Print and shaded views of the part. All mm, measured from the part's lowest x, y and z. A direction names the side the tool comes from. Give positions to 0.01 mm unless a question says otherwise; leave off trailing zeros. Loops run counter-clockwise (first coordinate to the right, second up) from the corner with the lowest first, then second, coordinate; pieces in that order, holes last. Notation, with made-up numbers: (27, 25) -> (56, 25) arc R29 ccw to (56, 57) -> close; hole circle Ø7 at (70.5, -19.5). An arc over 180 degrees is marked (long way). Answer as a JSON object with one key per item and string values. Group by question number.
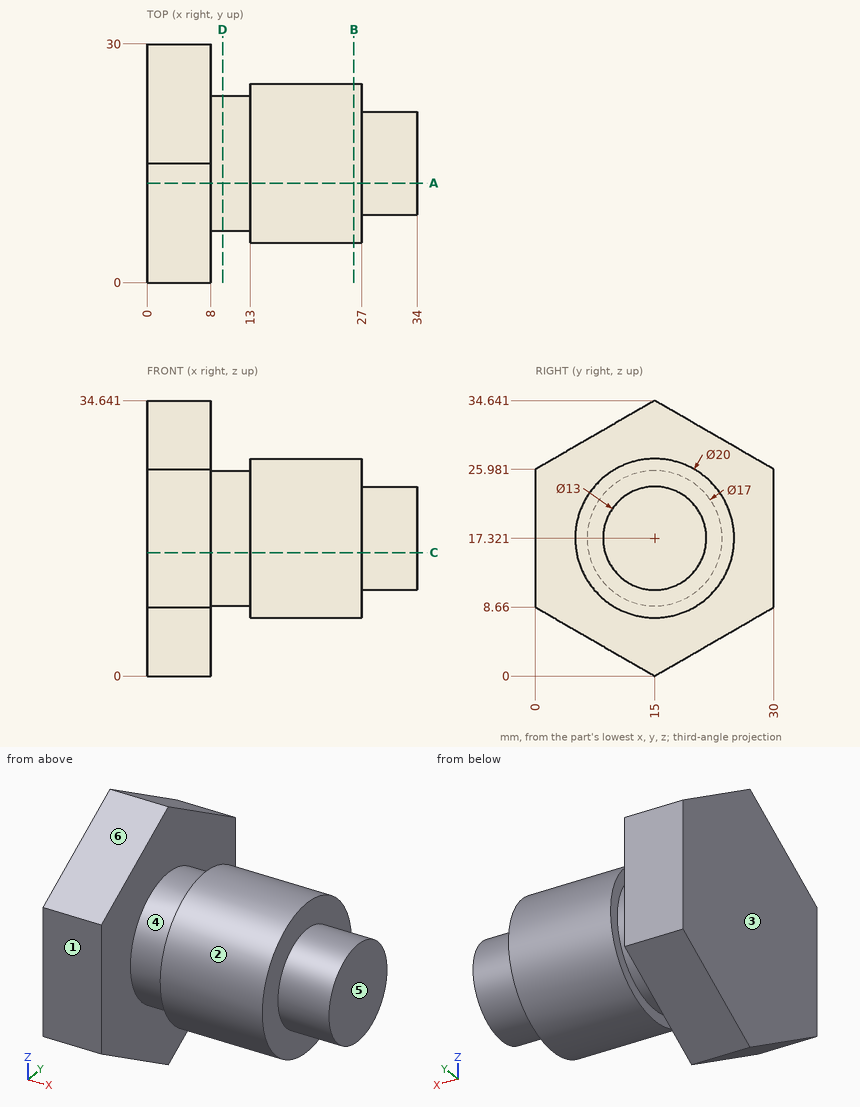
(1) Saw through at A-A on y = 12.5. List the corners of the cut face in (x, z) (1 decimal).
(2) Saw through at C-C on z = 15.5. List the corners of the cut face in (x, y).
(3) Pull direction X, two halves, no side cores. Call the marked faces 3, 4, 5 and 6: pulls with the +X half, pulls with the -X half, needs draft (parallel to the pull), parting line crosses it, or undercut.
(4) Saw through at D-D on x = 9.5. List the corners of the cut face in (y, z), plus the area to 3 significant figures.
(5) 3-axis set-ups, long thin cutter, end or side, ignore diameter. For the marked faces 1 and 2: which of +Z, -Z, +X, -X, +Y, -Y reach the whole face in a straight line?
(6) Probe line 1 along X through (y, z) = (6.5, 21); line 2 along X through (y, z) = (21.75, 16.5); line 3 along X through (y, z) = (15.25, 30.5). List the from-to ranges inside material, lowest first. Write a range as [from, to].
(7) Pin check, flat tips, straight feed: pin 1 (4 mm diameter, centred on y = 15.5, z = 29.5, fed in from +X); pin 2 (1.5 mm diameter, centred on x = 26, y = 21.5, fed in from -Z); pin 3 (2 mm diameter, centred on y = 14, z = 26.5, fed in from +X). Stop position of each tip, or through.
(8) Saw through at B-B on x = 26. List the corners of the cut face in (y, z).
Calculated:
{
 "1": {"outline": "(0, 1.4) -> (8, 1.4) -> (8, 9.2) -> (13, 9.2) -> (13, 7.6) -> (27, 7.6) -> (27, 11.3) -> (34, 11.3) -> (34, 23.3) -> (27, 23.3) -> (27, 27) -> (13, 27) -> (13, 25.4) -> (8, 25.4) -> (8, 33.2) -> (0, 33.2) -> close"},
 "2": {"outline": "(0, 0) -> (8, 0) -> (8, 6.7) -> (13, 6.7) -> (13, 5.17) -> (27, 5.17) -> (27, 8.76) -> (34, 8.76) -> (34, 21.24) -> (27, 21.24) -> (27, 24.83) -> (13, 24.83) -> (13, 23.3) -> (8, 23.3) -> (8, 30) -> (0, 30) -> close"},
 "3": {"face 3": "pulls with the -X half", "face 4": "undercut", "face 5": "pulls with the +X half", "face 6": "needs draft"},
 "4": {"outline": "circle Ø17 at (15, 17.32)", "area": "227 mm^2"},
 "5": {"face 1": "+Z, -Z, +X, -X, -Y", "face 2": "+X"},
 "6": {"line 1": "x = [0, 8], [13, 27]", "line 2": "x = [0, 27]", "line 3": "x = [0, 8]"},
 "7": {"pin 1": "stops at x = 8", "pin 2": "stops at z = 9.14", "pin 3": "stops at x = 27"},
 "8": {"outline": "circle Ø20 at (15, 17.32)"}
}
